Input: part model. Units: mm. Frame: model coordinates. A direction names the side the tool comes from. Coordinates: 2 decimals unless noted, no trailing zeros. Order: outer loops, then holes, each group sorted by start corner. A loop starts at its lowest first (then second) coordinate and runs counter-clockwise, first axis right, second up.
from build123d import *

# Parameters (mm, degrees)
SKETCH_R          = 42.5
PAD_DEPTH         = 70
THICKNESS_T       = -5
SKETCH001_R       = 15
POCKET_DEPTH      = 50
POCKET_DEPTH_BACK = -50
SKETCH002_W       = 2
SKETCH002_H       = 3


with BuildPart() as part:
    # Sketch → Pad (new body)
    with BuildSketch(Plane.XY):
        Circle(SKETCH_R)
    extrude(amount=PAD_DEPTH)

    # Thickness
    thickness_openings = [part.faces().sort_by_distance(p)[0] for p in [
        (0, 0, 0),
    ]]
    offset(amount=THICKNESS_T, openings=thickness_openings)

    # Sketch001 → Pocket (cut, two sides)
    with BuildSketch(Plane.YZ) as pocket_sk:
        with Locations((0, 30)):
            Circle(SKETCH001_R)
    extrude(amount=-POCKET_DEPTH, mode=Mode.SUBTRACT)
    extrude(pocket_sk.sketch, amount=-POCKET_DEPTH_BACK, mode=Mode.SUBTRACT)

    # Sketch002 → Groove (revolve, cut)
    with BuildSketch(Plane.XZ):
        with Locations((41.5, 61.5)):
            Rectangle(SKETCH002_W, SKETCH002_H)
        with Locations((41.5, 53.5)):
            Rectangle(SKETCH002_W, SKETCH002_H)
    revolve(axis=Axis((0, 0, 0), (0, 0, 1)), mode=Mode.SUBTRACT)


solid = part.part
Item 1: Draft query along Z for faces 4 (the face through (0, -38, 0)), 5 (the face through (-1, 1, 70)), 6 (the face through (-38, -16, 60)). Return one class per face: pulls with the +Z half, pulls with the -Z half, needs draft (parallel to the pull), parting line crosses it, or undercut.
Response values:
face 4: pulls with the -Z half
face 5: pulls with the +Z half
face 6: undercut
Item 2: Cut plane C-C on x = 0. Return loops of the section in (y, z).
Response values:
outline: (-42.5, 0) - (-37.5, 0) - (-37.5, 65) - (37.5, 65) - (37.5, 0) - (42.5, 0) - (42.5, 52) - (40.5, 52) - (40.5, 55) - (42.5, 55) - (42.5, 60) - (40.5, 60) - (40.5, 63) - (42.5, 63) - (42.5, 70) - (-42.5, 70) - (-42.5, 63) - (-40.5, 63) - (-40.5, 60) - (-42.5, 60) - (-42.5, 55) - (-40.5, 55) - (-40.5, 52) - (-42.5, 52) - close
Item 3: Access query for faces 1 (the face through (39.26, -16.28, 25.64)), 2 (the face through (17.3, -33.27, 32.04)), 3 (the face through (21.77, 34.15, 53.52)). Directions: +Z, -Z, +X, -X, +Y, -Y. A direction counts if a zero-diameter tool reaches every point of the face in a straight line with its end or side. Return the directions, or none.
Response values:
face 1: +Z, -Z
face 2: -Z
face 3: none
Item 4: Pin query (flat end, axial travel): pin 1 Ø8 at (x, z) = (-21, 56.5) entering from +Y; pin 2 Ø4 at (y, z) = (-17, 33.5) entering from +X; pin 3 Ø5 at (y, z) = (-11.5, 58.5) entering from -X. Return the tip coordinate at first contact, or that it passes through.
Response values:
pin 1: stops at y = 38.95
pin 2: stops at x = 39.76
pin 3: stops at x = -41.54
Item 5: Cut plane B-B on z = 30. Return loops of the section in (x, y).
Response values:
outline: (-39.76, -15) arc R42.5 ccw to (39.76, -15) - (34.37, -15) arc R37.5 cw to (-34.37, -15) - close; (-39.76, 15) - (-34.37, 15) arc R37.5 cw to (34.37, 15) - (39.76, 15) arc R42.5 ccw to start
Item 6: Cut plane A-A on y = 0. Count the separate pieces of the cut face and the enclosed holes in it, then the cut area to 3 significant figures.
Response values:
separate pieces: 3
enclosed holes: 0
area: 751 mm2
Item 7: Ray query, probe 1 along Z at (x, y) = (38.5, 0); probe 2 along Y at (x, z) = (0, 44); probe 3 along Z at (x, y) = (37, 0). Return the intervals inside material, ascending.
Response values:
probe 1: z = 0 to 15, 45 to 70
probe 2: y = -42.5 to -37.5, 37.5 to 42.5
probe 3: z = 65 to 70
Item 8: Cut plane D-D on z = 7. Return loops of the section in (x, y), then the cut area to 3 significant figures.
Response values:
outline: circle Ø85 at (0, 0); hole circle Ø75 at (0, 0)
area: 1,260 mm2
